from build123d import *

# Parameters (mm, degrees)
BOSS_EXTRUDE1_DEPTH     = 6
SKETCH3_W               = 6
SKETCH3_H               = 45
CUT_EXTRUDE1_DEPTH      = 1
CUT_EXTRUDE1_DEPTH_BACK = 7
FILLET1_R               = 5
CUT_EXTRUDE2_START      = -7
SKETCH4_R               = 1.5
CUT_EXTRUDE2_DEPTH      = 8


with BuildPart() as part:
    # Sketch1 → Boss-Extrude1 (new body)
    with BuildSketch(Plane.XY):
        Polygon((25, 0), (-25, 0), (-25, -25), (-18, -90), (18, -90), (25, -25), align=None)
    extrude(amount=BOSS_EXTRUDE1_DEPTH)

    # Sketch3 → Cut-Extrude1 (cut, two sides)
    with BuildSketch(Plane.XY.offset(6)) as cut_extrude1_sk:
        with Locations((0, -67.5)):
            Rectangle(SKETCH3_W, SKETCH3_H)
    extrude(amount=CUT_EXTRUDE1_DEPTH, mode=Mode.SUBTRACT)
    extrude(cut_extrude1_sk.sketch, amount=-CUT_EXTRUDE1_DEPTH_BACK, mode=Mode.SUBTRACT)

    # Fillet1
    fillet1_edges = [part.edges().sort_by_distance(p)[0] for p in [
        (18, -90, 3),
        (-18, -90, 3),
    ]]
    fillet(fillet1_edges, radius=FILLET1_R)

    # Sketch4 → Cut-Extrude2 (cut)
    with BuildSketch(Plane(origin=(0, 0, 0), x_dir=(-1, 0, 0), z_dir=(0, 0, -1)).offset(CUT_EXTRUDE2_START)):
        with Locations((-12.5, -20)):
            Circle(SKETCH4_R)
    cut_extrude2 = extrude(amount=CUT_EXTRUDE2_DEPTH, mode=Mode.SUBTRACT)

    # Mirror1: Cut-Extrude2 across plane
    add(cut_extrude2.mirror(Plane(origin=(0, 0, 0), x_dir=(0, 0, 1), z_dir=(1, 0, 0))), mode=Mode.SUBTRACT)


solid = part.part
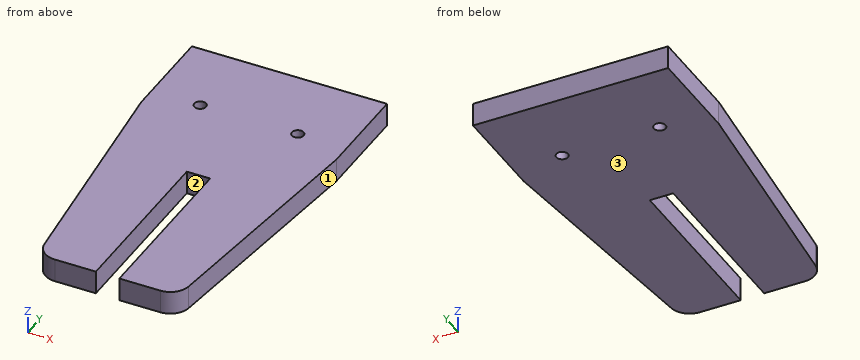
Work out the finished part from the listing and answer in its coordinate system (mm). Face numbers are marked on the shaded views. Give positions to 0.01 mm unless a question says otherwise; leave off trailing zeros. Order: outer loops, then holes, each group sorted by start corner. A loop starts at its lowest first (then second) coordinate and runs counter-clockwise, first axis right, second up. Notation, with made-up numbers: (29, 74) -> (85, 74) arc R26 ccw to (85, 102) -> close; hole circle Ø10 at (-9, 84). An arc over 180 degrees is marked (long way). Answer as a JSON object with one key per item and string values. Group by question number.
1. Section A-A on y = -20 is taken. Determine the outline of the cut face in (x, z), plus the area to 3 significant figures.
2. The mould has two halves that part along X. Classify the marked faces 1, 2 and 3: released by +X, released by -X, zero draft, split by the parting line, or undercut.
3. Section B-B on x = -12.5 is taken. Determine the outline of the cut face in (y, z).
4. Flat-ended cylindrical pins translate along their axes: pin 1 Ø1.8 at (x, z) = (1, 3) entering from -Y; pin 2 Ø1.5 at (y, z) = (-28, 1) entering from +X. Find the tip coordinate at first contact, or state that the pin passes through.
5. Section C-C on z = 1.25 is taken. Determine the outline of the cut face in (x, y).
6. Consider line 1 along Y through (x, z) = (12.5, 3.1); line 2 along X through (y, z) = (-50, 5.75); line 3 along X through (y, z) = (-46, 4.65). Determine where each line is inside the solid, lowest interval first. Write a range as [from, to].
7. Section D-D on y = -80 is taken. Determine the outline of the cut face in (x, z), plus the area to 3 significant figures.
Result sheet:
{
 "1": {"outline": "(-25, 0) -> (-14, 0) -> (-14, 6) -> (-25, 6) -> close; (-11, 0) -> (11, 0) -> (11, 6) -> (-11, 6) -> close; (14, 0) -> (25, 0) -> (25, 6) -> (14, 6) -> close", "area": "264 mm^2"},
 "2": {"face 1": "released by +X", "face 2": "undercut", "face 3": "zero draft"},
 "3": {"outline": "(-90, 0) -> (-21.5, 0) -> (-21.5, 6) -> (-90, 6) -> close; (-18.5, 0) -> (0, 0) -> (0, 6) -> (-18.5, 6) -> close"},
 "4": {"pin 1": "stops at y = -45", "pin 2": "stops at x = 24.76"},
 "5": {"outline": "(-25, -25) -> (-18.48, -85.54) arc R5 ccw to (-13.51, -90) -> (-3, -90) -> (-3, -45) -> (3, -45) -> (3, -90) -> (13.51, -90) arc R5 ccw to (18.48, -85.54) -> (25, -25) -> (25, 0) -> (-25, 0) -> close; hole circle Ø3 at (-12.5, -20); hole circle Ø3 at (12.5, -20)"},
 "6": {"line 1": "y = [-90, -21.5], [-18.5, 0]", "line 2": "x = [-22.31, -3], [3, 22.31]", "line 3": "x = [-22.74, -3], [3, 22.74]"},
 "7": {"outline": "(-19.08, 0) -> (-3, 0) -> (-3, 6) -> (-19.08, 6) -> close; (3, 0) -> (19.08, 0) -> (19.08, 6) -> (3, 6) -> close", "area": "193 mm^2"}
}
